Input: part model. Units: mm. Frame: model coordinates. Round coordinates to 2 decimals unless told otherwise and drop trailing zeros. Use one line per item in the form item = value. Start each with the question number.
Q1. Section query A-A, the plane x = -34.5. State how many separate pieces and enclosed holes the cut face has, and give its area (3 significant figures).
Q2. First-contact query: P1, Ø1, axis at x = -11, z = 37, coming from the +Y side; P2, Ø0.6, axis at y = -1, z = -14.5, coming from the -X side. Flat tips, straight axial feed; report the tip coordinate or a pass-through.
Q3. Ray query, line 1 along X through (y, z) = (-0.25, 38); line 2 along X through (y, z) = (-1.5, -28); line 3 along X through (y, z) = (-1.75, 9). Return the intervals inside material, ascending.
```python
from build123d import *

# Parameters (mm, degrees)
F0_W     = 50.984893
F0_H     = 2.100501
F0_W_2   = 50.602986
F0_H_2   = 2.482414
F0_W_3   = 51.175848
F0_H_3   = 2.86432
F0_H_4   = 3.246229
F0_W_4   = 50.412029
F0_W_5   = 50.221075
F0_W_6   = 50.030118
F0_H_5   = 2.673368
F0_W_7   = 49.839167
F0_H_6   = 2.864324
F1_DEPTH = 2


with BuildPart() as f1:
    # F0 (on Front) → F1 (new body)
    with BuildSketch(Plane.XZ):
        Polygon((-48.025098, -41.532639), (-48.025098, -55.854235), (47.834139, -55.854235), (47.834139, -41.532639), (12.698486, -41.532639), (12.698486, -38.859274), (47.834139, -38.859274), (47.834139, -29.120585), (12.698486, -29.120585), (12.698486, -26.06531), (47.834139, -26.06531), (47.834139, -16.326623), (12.125621, -16.326623), (12.125621, -12.889439), (47.834139, -12.889439), (47.834139, -3.91457), (12.125621, -3.91457), (12.125621, -1.43216), (47.834139, -1.43216), (47.834139, 8.497482), (12.125621, 8.497482), (12.125621, 11.552757), (47.834139, 11.552757), (47.834139, 20.71858), (12.125621, 20.71858), (12.125621, 23.5829), (47.834139, 23.5829), (47.834139, 31.030132), (12.125621, 31.030132), (12.125621, 33.703495), (47.834139, 33.703495), (47.834139, 66.356741), (-48.025098, 66.356741), (-48.025098, 33.703495), (-11.361802, 33.703495), (-11.361802, 30.457268), (-48.025098, 30.457268), (-48.025098, 22.819081), (-11.361802, 22.819081), (-11.361802, 19.763807), (-48.025098, 19.763807), (-48.025098, 10.979893), (-11.361802, 10.979893), (-11.361802, 7.924618), (-48.025098, 7.924618), (-48.025098, -1.43216), (-11.361802, -1.43216), (-11.361802, -4.29648), (-48.025098, -4.29648), (-48.025098, -12.889439), (-11.361802, -12.889439), (-11.361802, -16.326623), (-48.025098, -16.326623), (-48.025098, -26.06531), (-11.170847, -26.06531), (-11.170847, -29.120585), (-48.025098, -29.120585), (-48.025098, -38.859274), (-11.170847, -38.859274), (-11.170847, -41.532639), align=None)
        with Locations((2.291455, -46.783892)):
            Rectangle(F0_W, F0_H, mode=Mode.SUBTRACT)
        with Locations((2.100502, -33.989929)):
            Rectangle(F0_W_2, F0_H_2, mode=Mode.SUBTRACT)
        with Locations((2.386933, -21.195967)):
            Rectangle(F0_W_3, F0_H_3, mode=Mode.SUBTRACT)
        with Locations((2.291455, -8.592959)):
            Rectangle(F0_W, F0_H_4, mode=Mode.SUBTRACT)
        with Locations((2.005024, 3.437183)):
            Rectangle(F0_W_4, F0_H_4, mode=Mode.SUBTRACT)
        with Locations((1.909546, 15.276373)):
            Rectangle(F0_W_5, F0_H_4, mode=Mode.SUBTRACT)
        with Locations((1.814068, 27.401994)):
            Rectangle(F0_W_6, F0_H_5, mode=Mode.SUBTRACT)
        with Locations((1.718592, 37.236158)):
            Rectangle(F0_W_7, F0_H_6, mode=Mode.SUBTRACT)
    extrude(amount=F1_DEPTH)


solid = f1.part
```
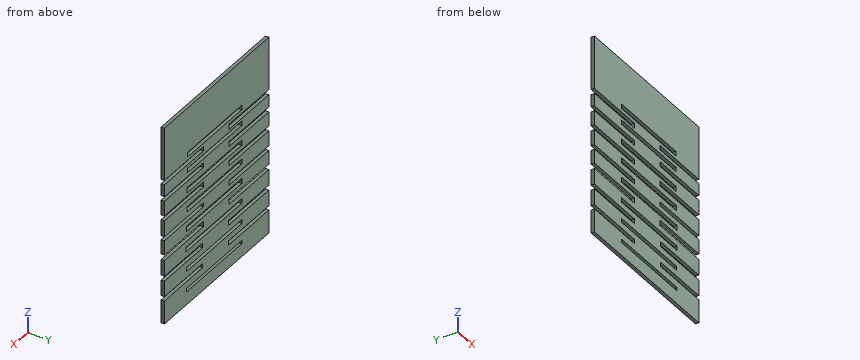
Results found:
q1.separate_pieces = 8
q1.enclosed_holes = 0
q1.area = 202 mm²
q2.P1 = through
q2.P2 = -11.36
q3.line_1 = -48.03 to -23.2, 26.64 to 47.83
q3.line_2 = -11.17 to 12.7
q3.line_3 = -11.36 to 12.13
